The model under review builds one solid part; all positions refer to its coordinate system, in mm. Face numbers are marked on the shaded views. A direction names the side the tool comes from. Round coordinates to 2 decimals unless told otherwise and drop trailing zeros. Order: outer loops, then holes, each group sorted by start corner. A loop starts at its lowest first (then second) coordinate and runs counter-clockwise, first axis right, second up.
from build123d import *

# Parameters (mm, degrees)
PAD_DEPTH    = 45
PAD001_DEPTH = 15


with BuildPart() as part:
    # Sketch001 → Pad (new body)
    with BuildSketch(Plane.XZ.offset(10)):
        Polygon((-40.888459, 65.334051), (-2.636269, 77.02892), (5.830902, 49.334051), (-40.888459, 49.334051), align=None)
        Polygon((20.506097, 48.790368), (48.790368, 20.506097), (60.104076, 31.819805), (31.819805, 60.104076), align=None)
    extrude(amount=PAD_DEPTH)

    # Sketch → Pad001 (new body)
    with BuildSketch(Plane.XZ.offset(55)):
        with BuildLine():
            ThreePointArc((40, 0), (15.122358, 37.031261), (-28.565714, 28))
            Line((-70, 28), (-28.565714, 28))
            Line((-70, 58), (-70, 28))
            Line((0, 58), (-70, 58))
            ThreePointArc((58, 0), (41.012193, 41.012193), (0, 58))
            Line((40, 0), (58, 0))
        make_face()
    extrude(amount=-PAD001_DEPTH)


solid = part.part
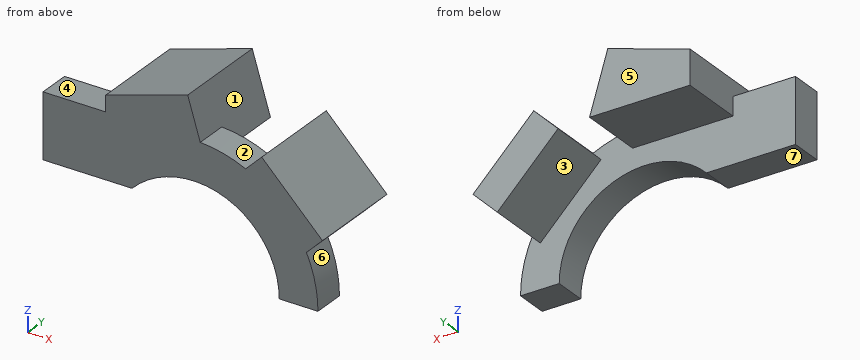
(1) We need section B-B (z = 54). Give the boundary of the cut face in (x, y).
(2) We need section A-A (y = -37.5). Give the boundary of the cut face in (x, z), and give its area (3 significant figures).
(3) Clearance check with flat-ended pins moving along their axes: P1, Ø4, axis at y = -42, z = 17.5, coming from the +X side; P2, Ø12, axis at y = -46.5, z = 67, coming from the -X side; P3, Ø16.5, axis at x = -62.5, y = -45.5, coming from the +Z side. State where each tip first meets the part, or that it passes through.
(4) We need section D-D (x = 1). Give the boundary of the cut face in (y, z).
(5) To check wall thickness, follow L1, parallel to Y at x = 8, z = 50; L2, parallel to X at y = -25.5, z = 27; L3, parallel to Z at x = 10, y = -43. State the ranges of each line that lie inside material, in increasing order.
(6) We need section C-C (y = -50.5). Give the boundary of the cut face in (x, z), and give its area (3 significant figures).
(7) Tool access review of the marked faces 1, 2, 3 and 4: name each direction out of +Z, -Z, +X, -X, +Y, -Y from which nothing blocks a thin tool from reaching the whole face with its end or side.
(8) The part is to be moulded in two halves that separate along Z. For the marked faces 5, 6 and 7, say which applies: pulls with the +Z half, pulls with the -Z half, needs draft (parallel to the pull), parting line crosses it, or undercut.
Verdict:
1. outline: (-70, -55) - (21.17, -55) - (21.17, -40) - (4.4, -40) - (4.4, -10) - (-40.89, -10) - (-40.89, -40) - (-70, -40) - close; (25.72, -55) - (37.92, -55) - (37.92, -10) - (25.72, -10) - close
2. outline: (-40.89, 49.33) - (5.83, 49.33) - (-2.64, 77.03) - (-40.89, 65.33) - close; (20.51, 48.79) - (48.79, 20.51) - (60.1, 31.82) - (31.82, 60.1) - close
2. area: 1,590 mm2
3. P1: stops at x = 55.89
3. P2: stops at x = -40.89
3. P3: stops at z = 58
4. outline: (-55, 39.99) - (-40, 39.99) - (-40, 49.33) - (-10, 49.33) - (-10, 65.14) - (-55, 65.14) - close
5. L1: y = -55 to -40
5. L2: x = 42.3 to 55.28
5. L3: z = 38.73 to 57.13
6. outline: (-70, 28) - (-28.57, 28) arc R40 cw to (40, 0) - (58, 0) arc R58 ccw to (52.64, 24.35) - (60.1, 31.82) - (31.82, 60.1) - (24.35, 52.64) arc R58 ccw to (3.21, 57.91) - (-2.64, 77.03) - (-40.89, 65.33) - (-40.89, 58) - (-70, 58) - close
6. area: 4,140 mm2
7. face 1: +Z, +Y
7. face 2: +Z, +Y, -Y
7. face 3: -Z, -X, +Y
7. face 4: +Z, -X, +Y, -Y
8. face 5: needs draft
8. face 6: undercut
8. face 7: pulls with the -Z half
